CAD build for the part. Positions are in the model's coordinates, mm. Face numbers are marked on the shaded views. A direction names the side the tool comes from. Round coordinates to 2 decimals unless told otherwise and drop trailing zeros. Loops run counter-clockwise (first coordinate to the right, second up) from the corner with the lowest first, then second, coordinate; pieces in that order, holes last. Notation, with made-up numbers: M 38,47.25 L 42,47.25 A13 cw 42,63.25 Z; hole C 22,79.5 d8. An arc over 180 degrees is marked long. Use one line per item in the form item = value.
Autodesk Inventor part; units mm, degrees
ref_plane "YZ Plane" through (0, 0, 0) normal (1, 0, 0) x (0, 1, 0)
ref_plane "XZ Plane" through (0, 0, 0) normal (0, 1, 0) x (-1, 0, 0)
ref_plane "XY Plane" through (0, 0, 0) normal (0, 0, 1) x (1, 0, 0)
sketch "Sketch1" plane through (0, 0, 0) normal (0, 1, 0) x (-1, 0, 0)
  circle A0 centre (0, 0) radius 317.5
  circle A1 centre (0, 0) radius 380.1959
  dimension "d0" = 635
  dimension "d1" = 760.3918
extrude "Extrusion1" add sketch "Sketch1" along normal blind 381
sketch "Sketch2" plane through (0, 0, 0) normal (0, -1, 0) x (1, 0, 0)
  line L0 (635, 635) -> (-635, 635)
  line L1 (-635, 635) -> (-635, -635)
  line L2 (-635, -635) -> (635, -635)
  line L3 (635, -635) -> (635, 635)
  circle A0 centre (0, 0) radius 380.1959
  dimension "d4" = 635
  dimension "d5" = 635
  dimension "d6" = 635
  dimension "d7" = 635
extrude "Extrusion2" add sketch "Sketch2" along normal blind 76.2 contours L3 L2 L1 L0 | A0
sketch "Sketch3" plane through (0, 381, 0) normal (0, 1, 0) x (1, 0, 0)
  circle A0 centre (0, 0) radius 349.7159
  circle A1 centre (0, 0) radius 380.1959
  circle A2 centre (0, 0) radius 317.5
  dimension "d10" = 30.48
  dimension "d11" = 760.3918
  dimension "d12" = 32.2159
extrude "Extrusion3" cut sketch "Sketch3" against normal blind 38.1 contours A0 | A2
properties part number "1"
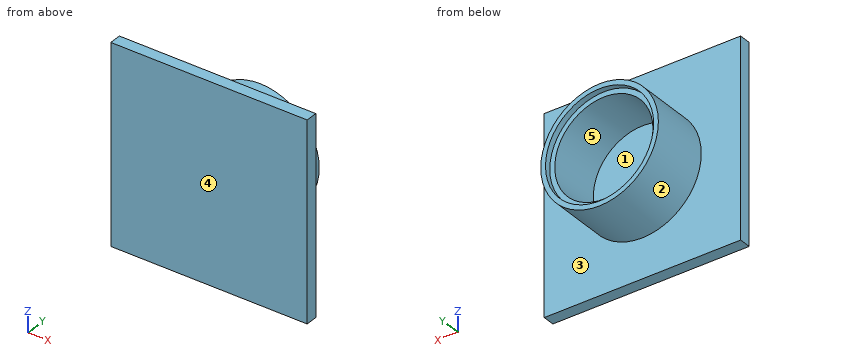
1. Cut at A-A on z = 0. Write the cut outline in (x, y), and give its area (3 significant figures).
Completed:
outline = M -635,-76.2 L 635,-76.2 L 635,0 L 380.2,0 L 380.2,381 L 349.72,381 L 349.72,342.9 L 317.5,342.9 L 317.5,0 L -317.5,0 L -317.5,342.9 L -349.72,342.9 L -349.72,381 L -380.2,381 L -380.2,0 L -635,0 Z
area = 142,000 mm2
2. Probe line 1 along Z through (x, y) = (-2, 314.5); line 2 along Z through (x, y) = (0, 362); line 3 along Y through (x, z) = (100, -14). List the from-to ranges inside material, lowest first. Write a range as from..to.
Completed:
line_1 = -380.19..-317.49, 317.49..380.19
line_2 = -380.2..-349.72, 349.72..380.2
line_3 = -76.2..0
3. Cut at D-D on z = -451.5. Write the cut outline in (x, y).
Completed:
outline = M -635,-76.2 L 635,-76.2 L 635,0 L -635,0 Z
4. Drop flat-ended pins along their axis: P1, Ø2, axis at x = 257, z = -388.5, coming from the +Y side; P2, Ø5, axis at y = 232, z = 314.5, coming from the -X side; P3, Ø2, axis at x = 56, y = 182.5, coming from the +Z side. Give the stop position or say it passes through.
Completed:
P1 = 0
P2 = -217.27
P3 = 376.2
5. Cut at C-C on y = 301.5. Write the cut outline in (x, z), and give its area (3 significant figures).
Completed:
outline = C 0,0 d760.39; hole C 0,0 d635
area = 137,000 mm2
6. Tool access for the marked faces 4 and 5: list every direction of +Z, -Z, +X, -X, +Y, -Y with a clear straight run to the whole face (end or side of a thin tool).
Completed:
face_4 = +Z, -Z, +X, -X, -Y
face_5 = +Y
7. Cut at B-B on x = 0. Write the cut outline in (y, z).
Completed:
outline = M -76.2,-635 L 0,-635 L 0,-380.2 L 381,-380.2 L 381,-349.72 L 342.9,-349.72 L 342.9,-317.5 L 0,-317.5 L 0,317.5 L 342.9,317.5 L 342.9,349.72 L 381,349.72 L 381,380.2 L 0,380.2 L 0,635 L -76.2,635 Z
8. Pull direction X, two halves, no side cores. Call the marked faces 1, 2 and 3: +X half, -X half, draft (parallel to the pull), parting line (faces both ways), or undercut.
Completed:
face_1 = undercut
face_2 = parting line
face_3 = draft
